Read the model definition and answer for the solid it produces. Units are mm, in the model's axes. A direction names the side the tool comes from. Coordinates: 2 decimals unless noted, no trailing zeros. Order: outer loops, then holes, each group sorted by start corner. A loop starts at its lowest first (then second) coordinate and runs counter-clockwise, first axis right, second up. Notation, with made-up numbers: M 60.25,-4.75 L 80.25,-4.75 A20 cw 80.25,19.25 Z; hole C 23.5,-38.5 d10. An arc over 180 degrees is marked long. Put each result on its own line as item: value.
from build123d import *

# Parameters (mm, degrees)
F0_W     = 25.4
F0_H     = 381
F1_DEPTH = 25.4
F2_R     = 6.35
F3_DEPTH = 38.1
F5_DEPTH = 25.401


with BuildPart() as f1:
    # F0 (on Front) → F1 (new body)
    with BuildSketch(Plane.XZ):
        Rectangle(F0_W, F0_H)
    extrude(amount=F1_DEPTH)

    # F2 (on face) → F3 (cut)
    with BuildSketch(Plane.XY.offset(190.5)):
        with Locations((0, -12.7)):
            Circle(F2_R)
    extrude(amount=-F3_DEPTH, mode=Mode.SUBTRACT)

    # F4 (on face) → F5 (cut, through all)
    with BuildSketch(Plane.XZ.offset(25.4)):
        with BuildLine():
            ThreePointArc((0, -95.24857), (-3.175, -98.42357), (0, -101.59857))
            Line((0, -101.59857), (0, -95.24857))
        make_face()
        with BuildLine():
            Line((0, -95.24857), (0, -101.59857))
            ThreePointArc((0, -101.59857), (2.245064, -100.668634), (3.175, -98.42357))
            ThreePointArc((3.175, -98.42357), (2.245064, -96.178506), (0, -95.24857))
        make_face()
    extrude(amount=-F5_DEPTH, mode=Mode.SUBTRACT)


solid = f1.part
Q1. Given pin 1 (2 mm diameter, centred on x = -0.5, z = 77.5, fed in from +Y); pin 2 (7.5 mm diameter, centred on x = 0, y = -12.7, fed in from +Z), each flat-ended and moving along its own axis, determine where each tip first touches the part or whether it passes through.
Answers below:
pin 1: stops at y = 0
pin 2: stops at z = 152.4
Q2. A tool of negligible diameter and unlimited length cuts with its end or side. For faces 1 (the face through (-3, -6.9, 190.5)), 2 (the face through (-1.38, -18.9, 171.72)), from which of +Z, -Z, +X, -X, +Y, -Y can it reach the whole face along a straight path? Write none if from no direction.
Answers below:
face 1: +Z, +X, -X, +Y, -Y
face 2: +Z
Q3. Consider line 1 along Y through (x, z) = (0, 163); line 2 along Z through (x, y) = (-0.25, -22.5); line 3 along Z through (x, y) = (-0.25, -8.5). Determine where each line is inside the solid, lowest interval first.
Answers below:
line 1: y = -25.4 to -19.05, -6.35 to 0
line 2: z = -190.5 to -101.59, -95.26 to 190.5
line 3: z = -190.5 to -101.59, -95.26 to 152.4
Q4. Find section A-A on y = -12.7. Write down the section's boundary in (x, z) (3 decimals).
Answers below:
outline: M -12.7,-190.5 L 12.7,-190.5 L 12.7,190.5 L 6.35,190.5 L 6.35,152.4 L -6.35,152.4 L -6.35,190.5 L -12.7,190.5 Z; hole C 0,-98.424 d6.35
Q5. For a pull along X with two mould halves and no side action, classify faces 3 (the face through (0, 0, 3)), 4 (the face through (0, -13, 152.4)), 5 (the face through (12.7, -13, -3)) as +X half, -X half, draft (parallel to the pull), parting line (faces both ways), or undercut.
Answers below:
face 3: draft
face 4: undercut
face 5: +X half
